Autodesk Inventor part; units mm, degrees
ref_plane "YZ Plane" through (0, 0, 0) normal (1, 0, 0) x (0, 1, 0)
ref_plane "XZ Plane" through (0, 0, 0) normal (0, 1, 0) x (-1, 0, 0)
ref_plane "XY Plane" through (0, 0, 0) normal (0, 0, 1) x (1, 0, 0)
sketch "Sketch1" plane through (0, 0, 0) normal (0, 0, 1) x (1, 0, 0)
  line L0 (-17, 0) -> (-7, 0)
  line L1 (-7, 0) -> (-7, 0.5)
  line L2 (-7, 0.5) -> (7, 0.5)
  line L3 (7, 0.5) -> (7, 0)
  line L4 (7, 0) -> (17, 0)
  line L5 (17, 0) -> (17, 6)
  line L6 (17, 6) -> (16, 7)
  line L7 (16, 7) -> (16, 18)
  line L8 (16, 18) -> (9, 18)
  line L9 (9, 18) -> (5, 22)
  line L10 (5, 22) -> (-5, 22)
  line L11 (-5, 22) -> (-9, 18)
  line L12 (-9, 18) -> (-16, 18)
  line L13 (-16, 18) -> (-16, 7)
  line L14 (-16, 7) -> (-17, 6)
  line L15 (-17, 6) -> (-17, 0)
  line L16 (-23.8, 0) -> (23.8, 0) construction
  line L17 (0, -4.4) -> (0, 26.4) construction
  circle A0 centre (0, 11) radius 4
  line L18 (-7, 0.5) -> (-7, 20) construction
  point P0 (0, 0)
  point P1 (0, 22)
  point P2 (0, 0.5)
  dimension "d0" = 34
  dimension "d1" = 14
  dimension "d2" = 6
  dimension "d3" = 18
  dimension "d5" = 11
  dimension "d6" = 8
  dimension "d7" = 0.5
  dimension "d8" = 45
  dimension "d9" = 45
  dimension "d10" = 1
  dimension "d11" = 1
  dimension "d12" = 6
  dimension "d13" = 45
  dimension "d33" = 22
extrude "Extrusion1" add sketch "Sketch1" along normal mid plane 30
sketch "Sketch2" plane through (0, 0, -15) normal (0, 0, -1) x (-1, 0, 0)
  circle A0 centre (0, 11) radius 4
  circle A1 centre (0, 11) radius 7.5
  point P0 (0, 0)
  dimension "d17" = 15
extrude "Extrusion2" cut sketch "Sketch2" against normal blind 2
mirror "Mirror1" about plane through (0, 0, 0) normal (0, 0, 1) of "Extrusion2"
sketch "Sketch3" plane through (7, 0, 15) normal (0, -1, 0) x (1, 0, 0)
  line L0 (10, -30) -> (10, 0) construction
  line L1 (0, 0) -> (10, 0) construction
  line L2 (0, -30) -> (0, 0) construction
  line L3 (10, -30) -> (0, -30) construction
  line L4 (-14, -30) -> (-14, 0) construction
  line L5 (-24, 0) -> (-14, 0) construction
  line L6 (-24, 0) -> (-24, -30) construction
  line L7 (-14, -30) -> (-24, -30) construction
  line L8 (5, -6) -> (-19, -6) construction
  line L9 (-19, -6) -> (-19, -24) construction
  line L10 (-19, -24) -> (5, -24) construction
  line L11 (5, -24) -> (5, -6) construction
  line L12 (5, -6) -> (-19, -24) construction
  line L13 (-19, -6) -> (5, -24) construction
  point P0 (-7, -15)
  dimension "d21" = 18
  dimension "d29" = 24
hole "Hole1" at (12, 0, -9) at (-12, 0, -9) at (12, 0, 9) at (-12, 0, 9) direction (0, 1, 0) diameter 3.242 end through all
chamfer "Chamfer1" distance 1 angle 45 4 edges at (12, 0, 10.621) (12, 0, -7.379) (-12, 0, 10.621) (-12, 0, -7.379)
ref_plane "Work Plane1" through (0, 0, 0) normal (0, 0, 1) x (1, 0, 0)
equation "\"d9\" = d8"
equation "\"d11\" = d10"
equation "\"d12\" = d2"
properties part number "cojinete lineal"
Geometry: final body of the model. Coordinates: model frame, mm. A direction names the side the tool comes from. Coordinates: 2 decimals unless noted, no trailing zeros. Order: outer loops, then holes, each group sorted by start corner. A loop starts at its lowest first (then second) coordinate and runs counter-clockwise, first axis right, second up.
1) First-contact query: P1, Ø4, axis at x = 0.5, z = 3, coming from the -Y side; P2, Ø9, axis at y = 12.5, z = 4, coming from the -X side; P3, Ø5, axis at x = -12, z = -9, coming from the -Y side. Flat tips, straight axial feed; report the tip coordinate or a pass-through.
Result sheet:
P1: stops at y = 0.5
P2: stops at x = -16
P3: stops at y = 0.12
2) Section A-A (z = 9). Give the number of separate pieces and of enclosed holes in the cut face, then the cut area to 3 significant figures.
Result sheet:
separate pieces: 3
enclosed holes: 1
area: 469 mm2
3) Section B-B (x = 0). Return loops of the section in (y, z), then the cut area to 3 significant figures.
Result sheet:
outline: (0.5, -15) - (3.5, -15) - (3.5, -13) - (7, -13) - (7, 13) - (3.5, 13) - (3.5, 15) - (0.5, 15) - close; (15, -13) - (18.5, -13) - (18.5, -15) - (22, -15) - (22, 15) - (18.5, 15) - (18.5, 13) - (15, 13) - close
area: 377 mm2
4) Section C-C (y = 7.5). Return loops of the section in (x, z).
Result sheet:
outline: (-16, -15) - (-6.63, -15) - (-6.63, -13) - (-1.94, -13) - (-1.94, 13) - (-6.63, 13) - (-6.63, 15) - (-16, 15) - close; (1.94, -13) - (6.63, -13) - (6.63, -15) - (16, -15) - (16, 15) - (6.63, 15) - (6.63, 13) - (1.94, 13) - close; hole circle Ø3.24 at (-12, -9); hole circle Ø3.24 at (-12, 9); hole circle Ø3.24 at (12, -9); hole circle Ø3.24 at (12, 9)
5) Draft query along Y for faces 1 (the flat face through (3, 8, 13)), 2 (the cylindrical face through (10.9, 9.62, -7.81)), 3 (the flat face through (16.5, 6.5, -0.2)). Return one class per face: released by +Y, released by -Y, zero draft, split by the parting line, or undercut.
Result sheet:
face 1: undercut
face 2: zero draft
face 3: released by +Y
6) Set-up query: faces 4 (the flat face through (13, 18, 0)), 5 (the flat face through (-16, 13, 0)), 6 (the flat face through (-3, 8, -13)). Return all of +Z, -Z, +X, -X, +Y, -Y with unobstructed straight access to the full face (end or side cutting, diameter ignored); none if empty.
Result sheet:
face 4: +Z, -Z, +X, +Y
face 5: +Z, -Z, -X, +Y
face 6: -Z
7) Ray query, probe 1 along Z at (x, y) = (-12, 5); probe 2 along Y at (x, z) = (0, 1); probe 3 along X at (y, z) = (11.25, 3.75). Return the intervals inside material, ascending.
Result sheet:
probe 1: z = -15 to -10.62, -7.38 to 7.38, 10.62 to 15
probe 2: y = 0.5 to 7, 15 to 22
probe 3: x = -16 to -3.99, 3.99 to 16
8) Section D-D (z = -3.5). Return loops of the section in (x, y), then the cut area to 3 significant figures.
Result sheet:
outline: (-17, 0) - (-7, 0) - (-7, 0.5) - (7, 0.5) - (7, 0) - (17, 0) - (17, 6) - (16, 7) - (16, 18) - (9, 18) - (5, 22) - (-5, 22) - (-9, 18) - (-16, 18) - (-16, 7) - (-17, 6) - close; hole circle Ø8 at (0, 11)
area: 588 mm2
